Geometry check sheet. Reference: the model listing, model coordinates, mm. Face numbers are marked on the shaded views. A direction names the side the tool comes from. Give positions to 0.01 mm unless a question says otherwise; leave off trailing zeros. Order: outer loops, then holes, each group sorted by start corner. A loop starts at its lowest first (then second) coordinate and runs counter-clockwise, first axis right, second up. Notation, with made-up numbers: M -15.5,31 L 40.5,31 A32 cw 40.5,61 Z; hole C 1.5,89.25 d2. An arc over 180 degrees is marked long. Put each result on its own line as item: value. Start each with the question number.
Q1. Access from +Z, -Z, +X, -X, +Y, -Y to the whole of each face (thin tool, end or side, straight path). Record for the marked faces 4 and 5.
Q2. Mould release check, pull along Y, two halves, no side actions. Record for the marked faces 1, 2 and 3: +Y half, -Y half, draft (parallel to the pull), parting line (faces both ways), or undercut.
Q3. Material ranges on L1, parallel to Z at x = -7, y = 0; L2, parallel to Z at x = -3.5, y = 3; L3, parallel to X at y = -10, z = -20, recorded low to high.
Q4. Section check B-B on x = 8. Record the cut outline in (y, z), then the cut area to 3 significant figures.
Q5. Section check A-A on z = 20. Record the cut outline in (x, y), then the cut area to 3 significant figures.
Q6. Section check C-C on z = -22. Record the cut outline in (x, y).
Q7. Section check D-D on y = -8. State how many separate pieces and enclosed holes the cut face has, then the cut area to 3 significant figures.
Q8. Go/stop test with flat-tipped pins: pin 1 (8 mm diameter, centred on x = 10, y = 13.5, fed in from -Z); pin 2 (10 mm diameter, centred on x = 5, y = -4.5, fed in from +Z); pin 3 (10 mm diameter, centred on x = 8.5, y = 13, fed in from +Z); pin 4 (1 mm diameter, centred on x = -8, y = -11.5, fed in from +Z). Record where each tip stops, or that it passes through.
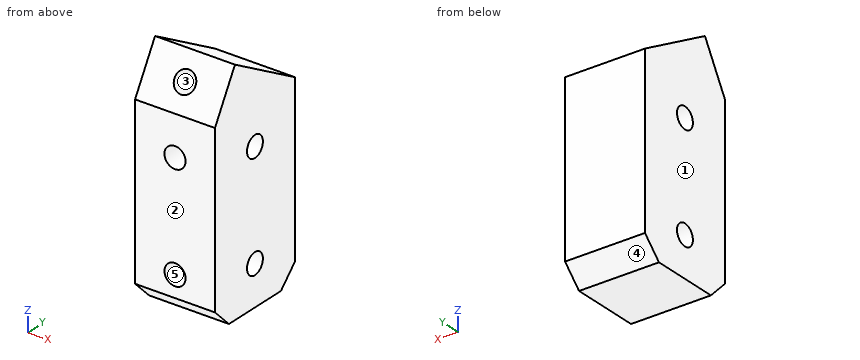
```python
from build123d import *

# Parameters (mm, degrees)
ESBO_O1_R                = 3.97
RESSALTO_EXTRUS_O1_DEPTH = 15
ESBO_O2_R                = 3.97
CORTE_EXTRUS_O2_DEPTH    = 20
CHANFRO1_SIZE            = 7
ESBO_O4_R                = 3.97
CORTE_EXTRUS_O4_DEPTH    = 20


with BuildPart() as part:
    # Esboço1 → Ressalto-extrusão1 (new body, symmetric)
    with BuildSketch(Plane(origin=(0, 0, 0), x_dir=(0, 0, -1), z_dir=(1, 0, 0))):
        Polygon((35, 20), (-35, 20), (-52.320508076, -10), (-35, -20), (35, -20), align=None)
        with Locations((-20, 0)):
            Circle(ESBO_O1_R, mode=Mode.SUBTRACT)
        with Locations((20, 0)):
            Circle(ESBO_O1_R, mode=Mode.SUBTRACT)
    extrude(amount=RESSALTO_EXTRUS_O1_DEPTH, both=True)

    # Esboço2 → Corte-extrusão2 (cut)
    with BuildSketch(Plane.XZ.offset(20)):
        with Locations((0, 20)):
            Circle(ESBO_O2_R)
        with Locations((0, -20)):
            Circle(ESBO_O2_R)
    extrude(amount=-CORTE_EXTRUS_O2_DEPTH, mode=Mode.SUBTRACT)

    # Chanfro1
    chanfro1_edges = [part.edges().sort_by_distance(p)[0] for p in [
        (0, 20, -35),
        (0, -20, -35),
    ]]
    chamfer(chanfro1_edges, length=CHANFRO1_SIZE)

    # Esboço4 → Corte-extrusão4 (cut)
    with BuildSketch(Plane(origin=(0, -30.155444566, 17.410254038), x_dir=(1, 0, 0), z_dir=(0, -0.866025404, 0.5))):
        with Locations((0, 30.310889132)):
            Circle(ESBO_O4_R)
    extrude(amount=-CORTE_EXTRUS_O4_DEPTH, mode=Mode.SUBTRACT)


solid = part.part
```
Results found:
1. face 4: -Z, +X, -X, +Y
1. face 5: -Y
2. face 1: draft
2. face 2: -Y half
2. face 3: undercut
3. L1: z = -35 to -23.97, -16.03 to 16.03, 23.97 to 46.55
3. L2: z = -35 to -22.6, -17.4 to 17.4, 22.6 to 34.84, 35.43 to 44.81
3. L3: x = -15 to -3.97, 3.97 to 15
4. outline: M -20,-28 L -13,-35 L 13,-35 L 20,-28 L 20,35 L -10,52.32 L -20,35 Z; hole C 0,-20 d7.94; hole C 0,20 d7.94
4. area: 3,000 mm^2
5. outline: M -15,-20 L -3.97,-20 L -3.97,-3.97 L -15,-3.97 Z; M -15,3.97 L 15,3.97 L 15,20 L -15,20 Z; M 3.97,-20 L 15,-20 L 15,-3.97 L 3.97,-3.97 Z
5. area: 835 mm^2
6. outline: M -15,-20 L -3.43,-20 L -3.43,-3.43 L -15,-3.43 Z; M -15,3.43 L 15,3.43 L 15,20 L -15,20 Z; M 3.43,-20 L 15,-20 L 15,-3.43 L 3.43,-3.43 Z
7. separate pieces: 1
7. enclosed holes: 3
7. area: 2,430 mm^2
8. pin 1: stops at z = -35
8. pin 2: stops at z = 52.03
8. pin 3: stops at z = 41.93
8. pin 4: stops at z = 50.59
